Build history of the part. All positions in model axes, mm. Face numbers are marked on the shaded views. A direction names the side the tool comes from. Round coordinates to 2 decimals unless told otherwise and drop trailing zeros. Write each loop counter-clockwise with the first axis right and the second up, starting at its lowest first coordinate (ties: lowest second). Pieces come first, ordered by that corner, then holes. Notation, with made-up numbers: (80.25, 59.5) -> (118.25, 59.5) arc R23 cw to (118.25, 96.5) -> close; hole circle Ø5 at (40, -8.5). An arc over 180 degrees is marked (long way). Answer in a Markdown table with one row per item. Add a question column.
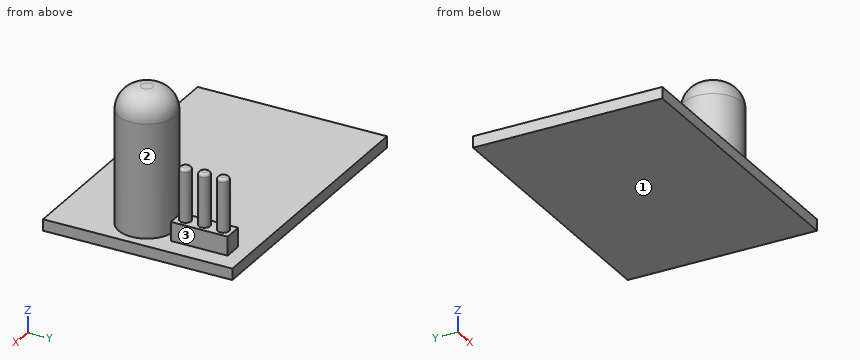
from build123d import *

# Parameters (mm, degrees)
SKIZZE1_W                       = 37
SKIZZE1_H                       = 25
AUFSATZ_LINEAR_AUSTRAGEN1_DEPTH = 1.5
SKIZZE3_R                       = 3.75
AUFSATZ_LINEAR_AUSTRAGEN2_DEPTH = 18
VERRUNDUNG1_R                   = 3
SKIZZE5_W                       = 2.5
SKIZZE5_H                       = 7.5
AUFSATZ_LINEAR_AUSTRAGEN3_DEPTH = 2.5
SKIZZE6_R                       = 0.75
AUFSATZ_LINEAR_AUSTRAGEN4_DEPTH = 7
LINEARES_MUSTER1_COUNT          = 3
LINEARES_MUSTER1_PITCH          = 2.5
VERRUNDUNG2_R                   = 0.4


with BuildPart() as part:
    # Skizze1 → Aufsatz-Linear austragen1 (new body)
    with BuildSketch(Plane.XY):
        Rectangle(SKIZZE1_W, SKIZZE1_H)
    extrude(amount=AUFSATZ_LINEAR_AUSTRAGEN1_DEPTH)

    # Skizze3 → Aufsatz-Linear austragen2 (add)
    with BuildSketch(Plane.XY.offset(1.5)):
        with Locations((13.564667913, -1.5)):
            Circle(SKIZZE3_R)
    extrude(amount=AUFSATZ_LINEAR_AUSTRAGEN2_DEPTH)

    # Verrundung1
    verrundung1_edges = [part.edges().sort_by_distance(p)[0] for p in [
        (9.814667913, -1.5, 19.5),
    ]]
    fillet(verrundung1_edges, radius=VERRUNDUNG1_R)



with BuildPart() as body_2:
    # Skizze5 → Aufsatz-Linear austragen3 (new body)
    with BuildSketch(Plane.XY.offset(1.5)):
        with Locations((14.75, 6.75)):
            Rectangle(SKIZZE5_W, SKIZZE5_H)
    extrude(amount=AUFSATZ_LINEAR_AUSTRAGEN3_DEPTH)


with BuildPart() as part_1:
    add(part.part)

    add(body_2.part)  # Aufsatz-Linear austragen4 merges body 2
    # Skizze6 → Aufsatz-Linear austragen4 (add)
    with BuildSketch(Plane.XY.offset(4)):
        with Locations((14.75, 9.25)):
            Circle(SKIZZE6_R)
    aufsatz_linear_austragen4 = extrude(amount=AUFSATZ_LINEAR_AUSTRAGEN4_DEPTH)

    # Lineares Muster1: Aufsatz-Linear austragen4 ×3
    with Locations(*[(0, -i * LINEARES_MUSTER1_PITCH, 0) for i in range(1, LINEARES_MUSTER1_COUNT)]):
        add(aufsatz_linear_austragen4)

    # Verrundung2
    verrundung2_edges = [part_1.edges().sort_by_distance(p)[0] for p in [
        (14, 9.25, 11),
        (14, 6.75, 11),
        (14, 4.25, 11),
    ]]
    fillet(verrundung2_edges, radius=VERRUNDUNG2_R)


solid = part_1.part
(1) Saw through at A-A (z = 3). List the corners of the cut face in (x, y), plus the area to 3 significant figures.
(2) Saw through at D-D (y = -7.5). List the corners of the cut face in (x, z).
(3) Which spindle directions (+Z, -Z, +X, -X, +Y, -Y) get a long thin tool onto all of the face, cutting with end or side? Do the marked faces 1, 2 and 3. Say none if no direction does.
(4) Saw through at C-C (z = 15). List the corners of the cut face in (x, y).
(5) Drop flat-ended pins along their axis: P1, Ø0.8, axis at y = 6.5, z = 3, coming from the -X side; P2, Ø0.8, axis at x = 15, z = 3, coming from the -Y side; P3, Ø4, axis at y = 0.5, z = 12, coming from the -X side; P4, Ø10, axis at x = 8.5, y = 9.5, coming from the -Z side. Give the stop position or say it passes through.
(6) Probe line 1 along Z through (x, y) = (8.5, -3.25); line 2 along Z through (x, y) = (15, 7.5); line 3 along Y through (x, z) = (17, 13.5). List the from-to ranges inside material, lowest first.
(7) Saw through at B-B (x = 6). List the corners of the cut face in (y, z), plus the area to 3 significant figures.
Answer sheet:
| question | item | result |
|---|---|---|
| 1 | outline | circle Ø7.5 at (13.56, -1.5); (13.5, 3) -> (16, 3) -> (16, 10.5) -> (13.5, 10.5) -> close |
| 1 | area | 62.9 mm² |
| 2 | outline | (-18.5, 0) -> (18.5, 0) -> (18.5, 1.5) -> (-18.5, 1.5) -> close |
| 3 | face 1 | -Z, +X, -X, +Y, -Y |
| 3 | face 2 | +Z |
| 3 | face 3 | +Z, +X, +Y |
| 4 | outline | circle Ø7.5 at (13.56, -1.5) |
| 5 | P1 | stops at x = 13.5 |
| 5 | P2 | stops at y = -5.1 |
| 5 | P3 | stops at x = 9.81 |
| 5 | P4 | stops at z = 0 |
| 6 | line 1 | z = 0 to 1.5 |
| 6 | line 2 | z = 0 to 4 |
| 6 | line 3 | y = -3 to 0 |
| 7 | outline | (-12.5, 0) -> (12.5, 0) -> (12.5, 1.5) -> (-12.5, 1.5) -> close |
| 7 | area | 37.5 mm² |
